```python
from build123d import *

# Parameters (mm, degrees)
SKETCH_1_W                  = 45
SKETCH_1_H                  = 50
EXTRUDE_1_DEPTH             = 5
EXTRUDE_2_DEPTH             = 9
EXTRUDE_START               = -9
EXTRUDE_3_DEPTH             = 9
SKETCH_4_R                  = 13
CUT_EXTRUDE_1_DEPTH         = 9
CUT_EXTRUDE_START           = -9
SKETCH_5_R                  = 13
CUT_EXTRUDE_2_DEPTH         = 9
SKETCH_6_W                  = 45
SKETCH_6_H                  = 5
EXTRUDE_4_DEPTH             = 5
FILLET_1_R                  = 2.5
HOLE_WIZARD_C_1_D           = 5.8
HOLE_WIZARD_C_1_DEPTH       = 5
HOLE_WIZARD_C_1_CBORE_D     = 11
HOLE_WIZARD_C_1_CBORE_DEPTH = 0.5
HOLE_WIZARD_C_1_TIP         = 1.742495795
SKETCH_15_R                 = 15
CUT_EXTRUDE_3_DEPTH         = 8
CUT_EXTRUDE_START_2         = -8
SKETCH_16_R                 = 15
CUT_EXTRUDE_4_DEPTH         = 8


with BuildPart() as part:
    # 草图1 → 凸台-拉伸1 (new body)
    with BuildSketch(Plane(origin=(0, 0, 0), x_dir=(1, 0, 0), z_dir=(0, 1, 0))):
        with Locations((22.5, 25)):
            Rectangle(SKETCH_1_W, SKETCH_1_H)
    extrude(amount=EXTRUDE_1_DEPTH)

    # 草图2 → 凸台-拉伸2 (add)
    with BuildSketch(Plane(origin=(45, 0, 0), x_dir=(0, 0, -1), z_dir=(1, 0, 0))):
        with BuildLine():
            Line((0, 5), (0, 9.920540101))
            Line((0, 9.920540101), (47.883739104, 61.528943381))
            ThreePointArc((47.883739104, 61.528943381), (76.148210795, 62.587073829), (77.206341243, 34.322602138))
            Line((77.206341243, 34.322602138), (50, 5))
            Line((50, 5), (0, 5))
        make_face()
    extrude(amount=-EXTRUDE_2_DEPTH)

    # 草图3 → 凸台-拉伸3 (add)
    with BuildSketch(Plane.ZY.offset(EXTRUDE_START)):
        with BuildLine():
            Line((-50, 5), (0, 5))
            Line((0, 5), (0, 9.920540101))
            Line((0, 9.920540101), (-47.883739104, 61.528943381))
            ThreePointArc((-47.883739104, 61.528943381), (-76.148210795, 62.587073829), (-77.206341243, 34.322602138))
            Line((-77.206341243, 34.322602138), (-50, 5))
        make_face()
    extrude(amount=EXTRUDE_3_DEPTH)

    # 草图4 → 切除-拉伸1 (cut)
    with BuildSketch(Plane.ZY):
        with Locations((-62.545040174, 47.92577276)):
            Circle(SKETCH_4_R)
    extrude(amount=-CUT_EXTRUDE_1_DEPTH, mode=Mode.SUBTRACT)

    # 草图5 → 切除-拉伸2 (cut)
    with BuildSketch(Plane(origin=(45, 0, 0), x_dir=(0, 0, -1), z_dir=(1, 0, 0)).offset(CUT_EXTRUDE_START)):
        with Locations(Location((62.545040174, 47.92577276, 0), (0, 0, 180))):
            Circle(SKETCH_5_R)
    extrude(amount=CUT_EXTRUDE_2_DEPTH, mode=Mode.SUBTRACT)

    # 草图6 → 凸台-拉伸4 (add)
    with BuildSketch(Plane(origin=(0, 0, -50), x_dir=(-1, 0, 0), z_dir=(0, 0, -1))):
        with Locations((-22.5, 2.5)):
            Rectangle(SKETCH_6_W, SKETCH_6_H)
    extrude(amount=EXTRUDE_4_DEPTH)

    # 圆角1
    # the kernel refuses this fillet: 2.5 mm, written as the material it adds along each edge
    with BuildSketch(Plane(origin=(9, 5, -50), x_dir=(0, 0, -1), z_dir=(-1, 0, 0))) as fillet_1_piece_1:
        with BuildLine():
            CenterArc((5.650108918, -2.413992211), FILLET_1_R, 105.072647289, 117.783385174)
            Line((3.817446285, -4.114388539), (3.780793032, -4.148396465))
            Line((3.780793032, -4.148396465), (-0.036653253, -0.034007927))
            Line((-0.036653253, -0.034007927), (0, 0.05))
            ThreePointArc((0, 0.05), (2.5, 0.05), (4.986997822, 0.048279844))
            Line((4.986997822, 0.048279844), (5, 0))
        make_face()
    extrude(amount=9)
    with BuildSketch(Plane(origin=(45, 5, -50), x_dir=(0, 0.7330650534621563, -0.6801585310738415), z_dir=(-1, 0, 0))) as fillet_1_piece_2:
        with BuildLine():
            CenterArc((5.612583111, 2.5), FILLET_1_R, 152.216614826, 117.783385174)
            Line((3.400792655, 3.665325267), (3.356556846, 3.688631773))
            ThreePointArc((3.356556846, 3.688631773), (1.663743075, 1.86667056), (-0.036653253, 0.034007927))
            Line((-0.036653253, 0.034007927), (0, -0.05))
            Line((0, -0.05), (5.612583111, -0.05))
            Line((5.612583111, -0.05), (5.612583111, 0))
        make_face()
    extrude(amount=9)

    # 打孔尺寸(%根据六角头螺)栓 C 级的类型1
    with Locations(Plane(origin=(22.5, 5, -21), x_dir=(0, 0, 1), z_dir=(0, 1, 0))):
        with Locations((0, 0), (14, 0), (-14, 0)):
            CounterBoreHole(HOLE_WIZARD_C_1_D / 2, HOLE_WIZARD_C_1_CBORE_D / 2, HOLE_WIZARD_C_1_CBORE_DEPTH, depth=HOLE_WIZARD_C_1_DEPTH)
            with Locations((0, 0, -(HOLE_WIZARD_C_1_DEPTH + HOLE_WIZARD_C_1_TIP / 2))):  # 118° drill point
                Cone(0, HOLE_WIZARD_C_1_D / 2, HOLE_WIZARD_C_1_TIP, mode=Mode.SUBTRACT)

    # 草图15 → 切除-拉伸3 (cut)
    with BuildSketch(Plane.ZY):
        with Locations((-62.545040174, 47.92577276)):
            Circle(SKETCH_15_R)
    extrude(amount=-CUT_EXTRUDE_3_DEPTH, mode=Mode.SUBTRACT)

    # 草图16 → 切除-拉伸4 (cut)
    with BuildSketch(Plane(origin=(45, 0, 0), x_dir=(0, 0, -1), z_dir=(1, 0, 0)).offset(CUT_EXTRUDE_START_2)):
        with Locations(Location((62.545040174, 47.92577276, 0), (0, 0, 180))):
            Circle(SKETCH_16_R)
    extrude(amount=CUT_EXTRUDE_4_DEPTH, mode=Mode.SUBTRACT)


solid = part.part
```
Geometry: final body of the model. Coordinates: model frame, mm. A direction names the side the tool comes from. Round coordinates to 2 decimals unless told otherwise and drop trailing zeros. Order: outer loops, then holes, each group sorted by start corner. A loop starts at its lowest first (then second) coordinate and runs counter-clockwise, first axis right, second up. Notation, with made-up numbers: M 20.25,-12.5 L 31.25,-12.5 A31 cw 31.25,24.5 Z; hole C 68,3 d5. An arc over 180 degrees is marked long. Use one line per item in the form item = value. Start each with the question number.
Q1. Pin query (flat end, axial travel): pin 1 Ø21 at (y, z) = (47.93, -62.55) entering from +X; pin 2 Ø8 at (x, y) = (7.5, 60.5) entering from -Z; pin 3 Ø1.5 at (x, z) = (17.5, -19) entering from +Y; pin 4 Ø9.5 at (x, z) = (22.5, -21) entering from +Y. Return the tip coordinate at first contact, or that it passes through.
Q2. Cut plane C-C (y = 64). Return loops of the section in (x, z), and give its area (3 significant figures).
Q3. Cut plane A-A (y = 49). Return loops of the section in (x, z), and give its area (3 significant figures).
Q4. Access query for faces 5 (the face through (40.94, 57.05, -74.45)), 6 (the face through (40.563, 35.363, -23.607)), 7 (the face through (3.94, 48.59, -77.53)), 8 (the face through (20, 4.5, -33)), 9 (the face through (40.6, 62.9, -75.8)). Directions: +Z, -Z, +X, -X, +Y, -Y. A direction counts if a zero-diameter tool reaches every point of the face in a straight line with its end or side. Return the directions, or none.
Q5. Material intervals for line 1 (X direction, y = 35.5, z = -73); line 2 (X direction, y = 4, z = -7); line 3 (Z direction, x = 22.5, y = 3), sorted ascending. Write a range as [from, to].
Q6. Cut plane B-B (z = -7). Return loops of the section in (x, y).
Q7. Cut plane D-D (x = 5.5). Return loops of the section in (y, z), and give its area (3 significant figures).
Q8. Mould query, pull axis Z, two halves, no side actions, for faces 1 (the face through (4.563, 6.689, -53.258)), 2 (the face through (24.152, 4.754, -15.754)), 3 (the face through (0, 26, -42)), 4 (the face through (21.39, 2.22, -37.68)). Classes: +Z half, -Z half, draft (parallel to the pull), parting line (faces both ways), or undercut.
Geometry results:
q1.pin_1 = through
q1.pin_2 = -80.61
q1.pin_3 = 5
q1.pin_4 = 4.5
q2.outline = M 0,-74.45 L 9,-74.45 L 9,-50.64 L 0,-50.64 Z; M 36,-74.45 L 45,-74.45 L 45,-50.64 L 36,-50.64 Z
q2.area = 428 mm^2
q3.outline = M 0,-82.52 L 9,-82.52 L 9,-75.5 L 8,-75.5 L 8,-77.51 L 0,-77.51 Z; M 0,-47.58 L 8,-47.58 L 8,-49.59 L 9,-49.59 L 9,-36.26 L 0,-36.26 Z; M 36,-82.52 L 45,-82.52 L 45,-77.51 L 37,-77.51 L 37,-75.5 L 36,-75.5 Z; M 36,-49.59 L 37,-49.59 L 37,-47.58 L 45,-47.58 L 45,-36.26 L 36,-36.26 Z
q3.area = 302 mm^2
q4.face_5 = +X
q4.face_6 = +Z, +X, -X, +Y
q4.face_7 = -X
q4.face_8 = +Y
q4.face_9 = +X, -X
q5.line_1 = [0, 9], [36, 45]
q5.line_2 = [0, 19.6], [25.4, 45]
q5.line_3 = [-55, -37.9], [-32.1, -23.9], [-18.1, -9.9], [-4.1, 0]
q6.outline = M 0,0 L 19.6,0 L 19.6,4.5 L 17,4.5 L 17,5 L 9,5 L 9,17.47 L 0,17.47 Z; M 25.4,0 L 45,0 L 45,17.47 L 36,17.47 L 36,5 L 28,5 L 28,4.5 L 25.4,4.5 Z
q7.outline = M 0,-55 L 5,-55 A2.5 cw 9.11,-53.82 L 34.32,-77.21 A20 ccw 61.53,-47.88 L 9.92,0 L 0,0 Z; hole C 47.93,-62.55 d30
q7.area = 2,530 mm^2
q8.face_1 = -Z half
q8.face_2 = undercut
q8.face_3 = draft
q8.face_4 = undercut
